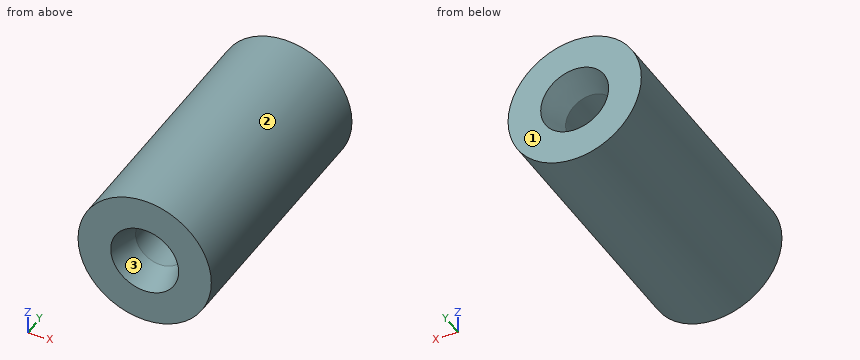
```python
from build123d import *

# Parameters (mm, degrees)
SKETCH1_R             = 5
BOSS_EXTRUDE1_DEPTH   = 19.5
SKETCH2_R             = 1.85
CUT_EXTRUDE1_DEPTH    = 26.5
CHAMFER1_SIZE         = 0.7
CHAMFER1_SIZE2        = 2.154378476
CHAMFER1_PART_2_SIZE  = 0.7
CHAMFER1_PART_2_SIZE2 = 2.154378476


with BuildPart() as part:
    # Sketch1 → Boss-Extrude1 (new body)
    with BuildSketch(Plane(origin=(0, 0, 0), x_dir=(1, 0, 0), z_dir=(0, 1, 0))):
        Circle(SKETCH1_R)
    extrude(amount=BOSS_EXTRUDE1_DEPTH)

    # Sketch2 → Cut-Extrude1 (cut)
    with BuildSketch(Plane(origin=(0, 19.5, 0), x_dir=(1, 0, 0), z_dir=(0, 1, 0))):
        Circle(SKETCH2_R)
    extrude(amount=-CUT_EXTRUDE1_DEPTH, mode=Mode.SUBTRACT)

    # Chamfer1
    chamfer1_edges = [part.edges().sort_by_distance(p)[0] for p in [
        (-1.85, 0, 0),
    ]]
    chamfer1_side = [part.faces().sort_by_distance(p)[0] for p in [
        (-4.858578644, 0, 0),
    ]]
    chamfer(chamfer1_edges, length=CHAMFER1_SIZE, length2=CHAMFER1_SIZE2, reference=chamfer1_side[0])

    # Chamfer1 part 2
    chamfer1_part_2_edges = [part.edges().sort_by_distance(p)[0] for p in [
        (-1.85, 19.5, 0),
    ]]
    chamfer1_part_2_side = [part.faces().sort_by_distance(p)[0] for p in [
        (-4.858578644, 19.5, 0),
    ]]
    chamfer(chamfer1_part_2_edges, length=CHAMFER1_PART_2_SIZE, length2=CHAMFER1_PART_2_SIZE2, reference=chamfer1_part_2_side[0])


solid = part.part
```
Check sheet for the modelled part. Datum: model origin and axes. Units: mm. Face numbers are marked on the shaded views. Round coordinates to 2 decimals unless told otherwise and drop trailing zeros. Order: outer loops, then holes, each group sorted by start corner. A loop starts at its lowest first (then second) coordinate and runs counter-clockwise, first axis right, second up. Notation, with made-up numbers: (70.5, 49.25) -> (93.5, 49.25) arc R8 ccw to (93.5, 54.25) -> close; hole circle Ø9 at (-2, -27). An arc over 180 degrees is marked (long way). One line per item, written item: value. Start each with the question number.
Q1. Gauge pin test, flat ends, axial feed: pin 1 Ø2 at (x, y) = (3, 16) entering from -Z; pin 2 Ø1 at (y, z) = (17.5, 3) entering from +X. Record the tip position at first contact, or that the pin passes through.
Q2. Cross-section at D-D (z = 4). Record the boundary of the cut face in (x, y).
Q3. Cross-section at A-A (x = 0). Record the boundary of the cut face in (y, z).
Q4. Thickness scan on line 1 (Z direction, x = 0, y = 13.5); line 2 (X direction, y = 12.5, z = 3). Record the ranges inside material, lowest first.
Q5. Cross-section at B-B (z = 0). Record the boundary of the cut face in (x, y), and give its area (3 significant figures).
Q6. Cross-section at C-C (y = 13). Record the boundary of the cut face in (x, z).
Q7. Mould release check, pull along X, two halves, no side actions. Record for the marked faces 1, 2 and 3: pulls with the +X half, pulls with the -X half, needs draft (parallel to the pull), parting line crosses it, or undercut.
Completed:
1. pin 1: stops at z = -4.58
1. pin 2: stops at x = 4.33
2. outline: (-3, 0) -> (3, 0) -> (3, 19.5) -> (-3, 19.5) -> close
3. outline: (0, -5) -> (19.5, -5) -> (19.5, -2.55) -> (17.35, -1.85) -> (2.15, -1.85) -> (0, -2.55) -> close; (0, 2.55) -> (2.15, 1.85) -> (17.35, 1.85) -> (19.5, 2.55) -> (19.5, 5) -> (0, 5) -> close
4. line 1: z = -5 to -1.85, 1.85 to 5
4. line 2: x = -4 to 4
5. outline: (-5, 0) -> (-2.55, 0) -> (-1.85, 2.15) -> (-1.85, 17.35) -> (-2.55, 19.5) -> (-5, 19.5) -> close; (1.85, 2.15) -> (2.55, 0) -> (5, 0) -> (5, 19.5) -> (2.55, 19.5) -> (1.85, 17.35) -> close
5. area: 120 mm²
6. outline: circle Ø10 at (0, 0); hole circle Ø3.7 at (0, 0)
7. face 1: needs draft
7. face 2: parting line crosses it
7. face 3: undercut
